Here's how the part is built. I have some questions about the finished solid (model axes, mm). Coordinates: 2 decimals unless noted, no trailing zeros. Order: outer loops, then holes, each group sorted by start corner. A loop starts at its lowest first (then second) coordinate and runs counter-clockwise, first axis right, second up. Notation, with made-up numbers: (22.5, 60) - (68.5, 60) arc R18 cw to (68.5, 65) - close; hole circle Ø8 at (10.25, 33.5). An arc over 180 degrees is marked (long way). Answer in a Markdown table with one row per item. Add a question column.
Item 1: I want a section at D-D (y = -29). Please give me the cut outline in (x, z), plus the area to 3 significant figures.
Item 2: Will these pins go through, and if not, where does the flat tip stop? pin 1 Ø6 at (y, z) = (-40.5, 19.5) entering from -X; pin 2 Ø12 at (x, z) = (-11, 48.5) entering from -Y; pin 3 Ø10 at (x, z) = (12.5, 13) entering from +Y.
Item 3: I want a section at B-B (z = 7.5). Please give me the cut outline in (x, y) (3 decimals), plus the area to 3 significant figures.
Item 4: Thinking about a two-plate mould opening in X: for faces 1 (the cylindrical face through (0.099, -22.225, 32.246)), 2 (the flat face through (0, -81, 0)), 3 (the flat face through (34.198, -82, 6)), which applies, +X half, -X half, draft (parallel to the pull), parting line (faces both ways), or undercut?
Item 5: I want a section at A-A (x = -17). Please give me the cut outline in (y, z).
Item 6: If I drill on line 1 along Y through (x, z) = (0, 11.5) (3 decimals); line 2 along X through (y, z) = (-48.5, 33); line 3 along Z through (x, y) = (-3, -33), over which ranges is the centre line in solid material (lowest first)? Write a range as from..to.
Item 7: I want a section at C-C (z = 32.5). Please give me the cut outline in (x, y) (3 decimals).
```python
from build123d import *

# Parameters (mm, degrees)
BOSS_EXTRUDE1_DEPTH  = 76.2
CUT_EXTRUDE1_START   = -34.198033
CUT_EXTRUDE1_DEPTH   = 68.396066318
M5_CLEARANCE_HOLE1_D = 5.5
CUT_EXTRUDE2_REACH   = 144.97
SKETCH10_R           = 19.05


with BuildPart() as part:
    # Sketch1 → Boss-Extrude1 (new body)
    with BuildSketch(Plane.XY):
        Polygon((34.198033159, -120.876287401), (34.198033159, -66.796344186), (0, -9.314618425), (-34.198033159, -66.796344186), (-34.198033159, -120.876287401), align=None)
    extrude(amount=BOSS_EXTRUDE1_DEPTH)

    # Sketch2 → Cut-Extrude1 (cut)
    with BuildSketch(Plane(origin=(0, 0, 0), x_dir=(0, 0, -1), z_dir=(1, 0, 0)).offset(CUT_EXTRUDE1_START)):
        with BuildLine():
            Line((-76.2, -120.876287401), (0, -120.876287401))
            ThreePointArc((0, -120.876287401), (-23.444492551, -62.806448146), (-68.2625, -19.067487592))
            Line((-68.2625, -19.067487592), (-68.2625, -9.314618425))
            Line((-68.2625, -9.314618425), (-76.2, -9.314618425))
            Line((-76.2, -9.314618425), (-76.2, -22.225))
            Line((-76.2, -22.225), (-76.2, -66.796344186))
            Line((-76.2, -66.796344186), (-76.2, -120.876287401))
        make_face()
    extrude(amount=CUT_EXTRUDE1_DEPTH, mode=Mode.SUBTRACT)

    # M5 Clearance Hole1 (through all)
    with Locations(Plane(origin=(0, 0, 0), x_dir=(-1, 0, 0), z_dir=(0, 0, -1))):
        with Locations((-15.875, -84.114050529), (15.875, -84.114050529), (0, -41.712872808)):
            Hole(M5_CLEARANCE_HOLE1_D / 2)

    # Sketch10 → Cut-Extrude2 (cut, up to next)
    with BuildSketch(Plane(origin=(0, 0, 0), x_dir=(-1, 0, 0), z_dir=(0, 0, -1)), mode=Mode.PRIVATE) as cut_extrude2_sk1:
        with Locations((0, -3.175)):
            Circle(SKETCH10_R)
    cut_extrude2_tool1 = extrude(cut_extrude2_sk1.sketch, amount=-CUT_EXTRUDE2_REACH, mode=Mode.PRIVATE) & part.part
    add(cut_extrude2_tool1.solids().sort_by_distance((0, -3.175, 0))[0], mode=Mode.SUBTRACT)


solid = part.part
```
Values follow:
| question | item | result |
|---|---|---|
| 1 | outline | (-11.71, 0) - (11.71, 0) - (11.71, 54.41) - (-11.71, 54.41) - close |
| 1 | area | 1,270 mm^2 |
| 2 | pin 1 | stops at x = -20.34 |
| 2 | pin 2 | stops at y = -39.68 |
| 2 | pin 3 | stops at y = -21.92 |
| 3 | outline | (-34.198, -93.711) - (34.198, -93.711) - (34.198, -66.796) - (6.909, -20.928) arc R19.05 cw to (-6.909, -20.928) - (-34.198, -66.796) - close; hole circle Ø5.5 at (-15.875, -84.114); hole circle Ø5.5 at (0, -41.713); hole circle Ø5.5 at (15.875, -84.114) |
| 3 | area | 3,640 mm^2 |
| 4 | face 1 | undercut |
| 4 | face 2 | draft |
| 4 | face 3 | +X half |
| 5 | outline | (-120.88, 0) - (-86.62, 0) - (-86.62, 10.39) arc R152.4 cw to start; (-81.6, 0) - (-37.89, 0) - (-37.89, 44.33) arc R152.4 cw to (-81.6, 12.69) - close |
| 6 | line 1 | y = -84.143..-44.463, -38.963..-22.225 |
| 6 | line 2 | x = -23.31..23.31 |
| 6 | line 3 | z = 0..49.65 |
| 7 | outline | (-24.594, -50.654) - (24.594, -50.654) - (6.909, -20.928) arc R19.05 cw to (-6.909, -20.928) - close; hole circle Ø5.5 at (0, -41.713) |
